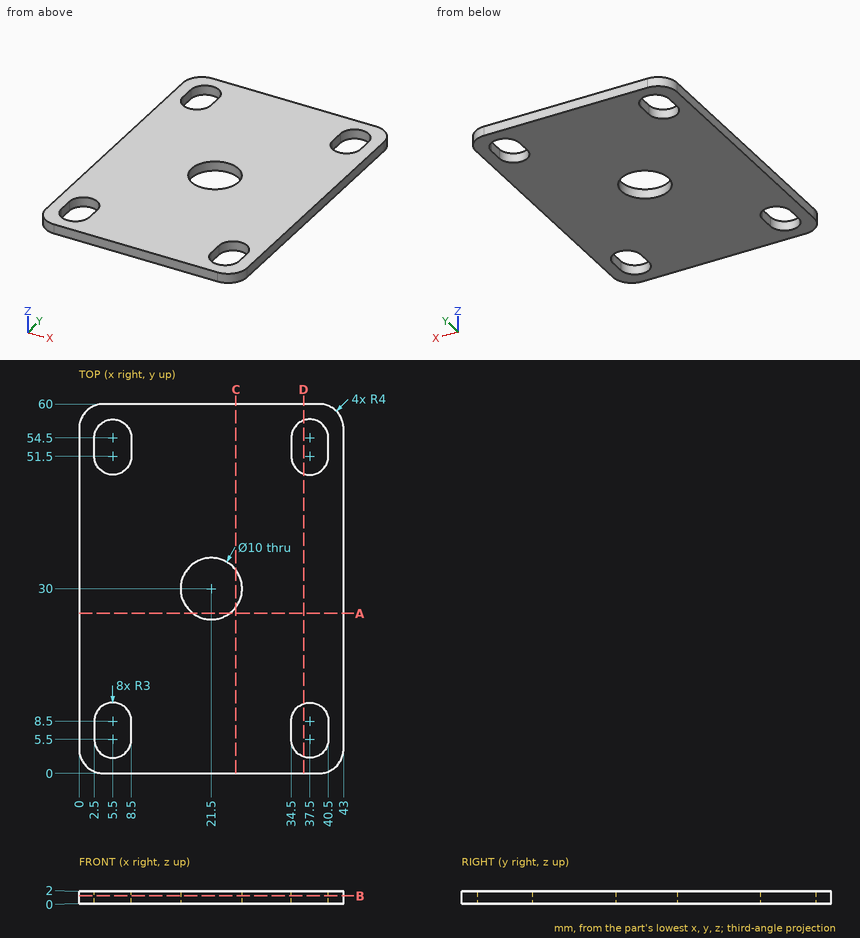
Source: three-view drawing plus pictorial views. Frame: mm from the lowest corner of the part. Give positions to 0.01 mm unless a question says otherwise; leave off trailing zeros. Order: outer loops, then holes, each group sorted by start corner. A loop starts at its lowest first (then second) coordinate and runs counter-clockwise, first axis right, second up. Notation, with made-up numbers: (-35, 52) -> (-11, 52) arc R19 ccw to (-11, 86) -> close; hole circle Ø8 at (78, -27.75). An arc over 180 degrees is marked (long way). Put each result on its own line as item: value.
Q1. Section C-C, the plane x = 25.5. Return loops of the section in (y, z).
Here are the results:
outline: (0, 0) -> (27, 0) -> (27, 2) -> (0, 2) -> close; (33, 0) -> (60, 0) -> (60, 2) -> (33, 2) -> close
Q2. Material intervals for L1, parallel to Y at x = 37.5, z = 0.3; L2, parallel to Y at x = 21.5, z = 1.1; L3, parallel to Y at x = 8, z = 1.05, sorted ascending.
Here are the results:
L1: y = 0 to 2.5, 11.5 to 48.5, 57.5 to 60
L2: y = 0 to 25, 35 to 60
L3: y = 0 to 3.84, 10.16 to 49.84, 56.16 to 60
Q3. Section D-D, the plane x = 36.5. Return loops of the section in (y, z).
Here are the results:
outline: (0, 0) -> (2.67, 0) -> (2.67, 2) -> (0, 2) -> close; (11.33, 0) -> (48.67, 0) -> (48.67, 2) -> (11.33, 2) -> close; (57.33, 0) -> (60, 0) -> (60, 2) -> (57.33, 2) -> close
Q4. Section B-B, the plane z = 1.25. Return loops of the section in (x, y).
Here are the results:
outline: (0, 4) arc R4 ccw to (4, 0) -> (39, 0) arc R4 ccw to (43, 4) -> (43, 56) arc R4 ccw to (39, 60) -> (4, 60) arc R4 ccw to (0, 56) -> close; hole (2.5, 5.5) arc R3 ccw to (8.5, 5.5) -> (8.5, 8.5) arc R3 ccw to (2.5, 8.5) -> close; hole (2.5, 51.5) arc R3 ccw to (8.5, 51.5) -> (8.5, 54.5) arc R3 ccw to (2.5, 54.5) -> close; hole circle Ø10 at (21.5, 30); hole (34.5, 5.5) arc R3 ccw to (40.5, 5.5) -> (40.5, 8.5) arc R3 ccw to (34.5, 8.5) -> close; hole (34.5, 51.5) arc R3 ccw to (40.5, 51.5) -> (40.5, 54.5) arc R3 ccw to (34.5, 54.5) -> close
Q5. Section A-A, the plane y = 26. Return loops of the section in (x, z).
Here are the results:
outline: (0, 0) -> (18.5, 0) -> (18.5, 2) -> (0, 2) -> close; (24.5, 0) -> (43, 0) -> (43, 2) -> (24.5, 2) -> close
